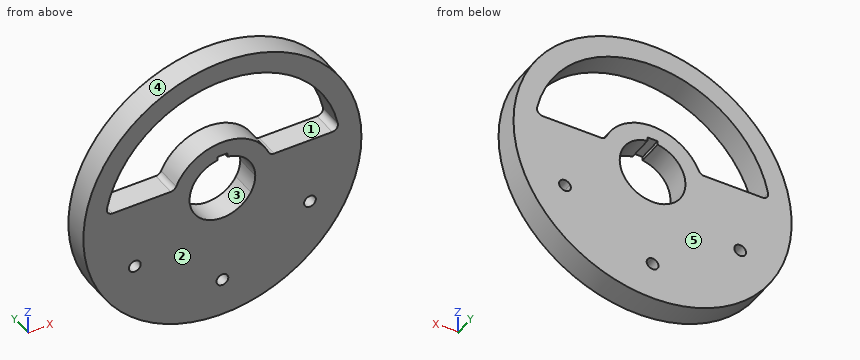
```python
from build123d import *

# Parameters (mm, degrees)
F0_R     = 82.5
F0_R_2   = 3.5
F1_DEPTH = 15
F2_R     = 3.5


with BuildPart() as f1:
    # F0 (on Front) → F1 (new body)
    with BuildSketch(Plane.XZ):
        Circle(F0_R)
        with Locations((-51.961524, -30)):
            Circle(F0_R_2, mode=Mode.SUBTRACT)
        with BuildLine():
            ThreePointArc((0, -56.5), (2.474874, -57.525126), (3.5, -60))
            ThreePointArc((3.5, -60), (-2.474874, -62.474874), (0, -56.5))
        make_face(mode=Mode.SUBTRACT)
        with BuildLine():
            ThreePointArc((55.461524, -30), (51.055658, -33.38074), (48.930435, -28.25))
            ThreePointArc((48.930435, -28.25), (52.867391, -26.61926), (55.461524, -30))
        make_face(mode=Mode.SUBTRACT)
        with BuildLine():
            ThreePointArc((19.5, 0), (18.835554, -5.046971), (16.887495, -9.75))
            ThreePointArc((16.887495, -9.75), (-16.084916, -11.02386), (-3, 19.267849))
            Line((-3, 19.267849), (-3, 21.5))
            Line((-3, 21.5), (0, 21.5))
            Line((0, 21.5), (3, 21.5))
            Line((3, 21.5), (3, 19.267849))
            ThreePointArc((3, 19.267849), (14.811313, 12.683651), (19.5, 0))
        make_face(mode=Mode.SUBTRACT)
        with BuildLine():
            Line((-28.284271, 10), (-69.282032, 10))
            ThreePointArc((-69.282032, 10), (0, 70), (69.282032, 10))
            Line((69.282032, 10), (28.284271, 10))
            ThreePointArc((28.284271, 10), (0, 30), (-28.284271, 10))
        make_face(mode=Mode.SUBTRACT)
    extrude(amount=F1_DEPTH)

    # F2
    f2_edges = [f1.edges().sort_by_distance(p)[0] for p in [
        (69.282032, -7.5, 10),
        (-69.282032, -7.5, 10),
        (-28.284271, -7.5, 10),
        (28.284271, -7.5, 10),
    ]]
    fillet(f2_edges, radius=F2_R)


solid = f1.part
```
Geometry: final body of the model. Coordinates: model frame, mm. Face numbers are marked on the shaded views. A direction names the side the tool comes from. Give positions to 0.01 mm unless a question says otherwise; leave off trailing zeros. Loops run counter-clockwise (first coordinate to the right, second up) from the corner with the lowest first, then second, coordinate; pieces in that order, holes last. Notation, with made-up numbers: (-7.75, 39.5) - (32.25, 39.5) arc R26 ccw to (32.25, 68.5) - close; hole circle Ø6 at (47, 54). An arc over 180 degrees is marked (long way). Answer as CSV lines item,"result". Start each with the question number.
(1) Pin query (flat end, axial travel): P1, Ø1, axis at y = -9, z = -2.5, coming from the +X side; P2, Ø0.7, axis at y = -5.5, z = 20.5, coming from the +X side; P3, Ø1, axis at y = -3, z = 32, coming from the -X side. Return the tip coordinate at first contact, or that it passes through.
(2) Reachability of the marked faces 1 and 2 from +Z, -Z, +X, -X, +Y, -Y: full face, straight path, thin tool, end or side. Return the list, or none.
(3) Section query C-C (y = -4.75). Output: boundary loops of the cut face in (x, z).
(4) Ray query, line 1 along Z through (x, y) = (7, -12); line 2 along Z through (x, y) = (16.5, -3.75); line 3 along X through (y, z) = (-7.25, -60). Return the intervals inside material, ascending. Write a range as [from, to].
(5) Section query B-B (z = 43). Output: boundary loops of the cut face in (x, y), and give its area (3 significant figures).
(6) Mould query, pull axis X, two halves, no side actions, for the marked faces 3, 4 and 5. Classes: +X half, -X half, draft (parallel to the pull), parting line (faces both ways), or undercut.
(7) Section query D-D (z = -50). Output: boundary loops of the cut face in (x, y), and give its area (3 significant figures).
(8) Section query A-A (x = -59). Output: boundary loops of the cut face in (y, z), and give its area (3 significant figures).
Worked answers:
1,P1,"stops at x = 82.48"
1,P2,"stops at x = 80"
1,P3,"stops at x = -76.25"
2,face 1,"+Y, -Y"
2,face 2,"+Z, -Z, +X, -X, -Y"
3,outline,"circle Ø165 at (0, 0); hole (-68.54, 14.21) arc R3.5 ccw to (-65.12, 10) - (-30.66, 10) arc R3.5 ccw to (-27.46, 12.09) arc R30 cw to (27.46, 12.09) arc R3.5 ccw to (30.66, 10) - (65.12, 10) arc R3.5 ccw to (68.54, 14.21) arc R70 ccw to start; hole circle Ø7 at (-51.96, -30); hole (-3, 19.27) arc R19.5 ccw (long way) to (16.89, -9.75) arc R19.5 ccw to (19.5, 0) arc R19.5 ccw to (3, 19.27) - (3, 21.5) - (-3, 21.5) - close; hole (0, -56.5) arc R3.5 ccw (long way) to (3.5, -60) arc R3.5 ccw to start; hole circle Ø7 at (51.96, -30)"
4,line 1,"z = [-82.2, -18.2], [18.2, 29.17], [69.65, 82.2]"
4,line 2,"z = [-80.83, -10.39], [10.39, 25.05], [68.03, 80.83]"
4,line 3,"x = [-56.62, -3.5], [3.5, 56.62]"
5,outline,"(-70.41, -15) - (-55.24, -15) - (-55.24, 0) - (-70.41, 0) - close; (55.24, -15) - (70.41, -15) - (70.41, 0) - (55.24, 0) - close"
5,area,"455 mm^2"
6,face 3,"undercut"
6,face 4,"parting line"
6,face 5,"draft"
7,outline,"(-65.62, -15) - (65.62, -15) - (65.62, 0) - (-65.62, 0) - close"
7,area,"1,970 mm^2"
8,outline,"(-15, -57.66) - (0, -57.66) - (0, 10) - (-15, 10) - close; (-15, 37.67) - (0, 37.67) - (0, 57.66) - (-15, 57.66) - close"
8,area,"1,310 mm^2"
